The listing builds one solid part. Answer for the finished solid, in the listing's coordinates (mm). Face numbers are marked on the shaded views. A direction names the side the tool comes from. Round coordinates to 2 decimals unless told otherwise and drop trailing zeros. Order: outer loops, then holes, each group sorted by start corner. A loop starts at its lowest first (then second) coordinate and runs counter-clockwise, first axis right, second up. Notation, with made-up numbers: M -29.5,-20.5 L 19.5,-20.5 A30 cw 19.5,4.5 Z; hole C 17.5,18 d1. An arc over 180 degrees is marked long. Write item = value, one per line. Start each with the question number.
(1) A cutting plane is placed at D-D, the plane x = -10. Determine the outline of the cut face in (y, z), and give its area (3 significant figures).
(2) A cutting plane is placed at B-B, the plane z = -0.5. Determine the outline of the cut face in (x, y).
(3) Straight lines are drawn through the part: probe 1 along Z at (x, y) = (-4, 4.3); probe 2 along X at (y, z) = (0.55, 15); probe 3 along X at (y, z) = (3.45, -7) (3 decimals). For each, find the intervals that lie inside material, in ascending order. Write a range as from..to.
(4) A cutting plane is placed at C-C, the plane y = 4.25. Count the separate pieces of the cut face and the enclosed holes in it, and give its area (3 significant figures).
(5) A cutting plane is placed at A-A, the plane x = 8.5. Determine the outline of the cut face in (y, z) (3 decimals), and give its area (3 significant figures).
(6) Each of these flat-tipped pins is pushed along its axis until it touches: pin 1 (1.7 mm diameter, centred on x = 10, z = 4.5, fed in from +Y); pin 2 (1.7 mm diameter, centred on x = -13.5, z = 15.5, fed in from +Y). Where does it stop, or does it pass through?
(7) Which of the six approach directions +Z, -Z, +X, -X, +Y, -Y give full straight-line access (tool end or side, diameter ignored) to the marked faces 1, 2 and 3?
from build123d import *

# Parameters (mm, degrees)
SKETCH1_W           = 45
SKETCH1_H           = 45
SKETCH1_R           = 1.7
BOSS_EXTRUDE1_DEPTH = 5
SKETCH7_R           = 2.9
CUT_EXTRUDE6_DEPTH  = 3
SKETCH4_R           = 0.925
CUT_EXTRUDE3_DEPTH  = 33.210246817
SKETCH5_R           = 0.95
CUT_EXTRUDE4_DEPTH  = 33.210246817
LPATTERN1_COUNT     = 5
LPATTERN1_PITCH     = 5
FILLET1_R           = 1
CUT_EXTRUDE7_START  = -4
CUT_EXTRUDE7_DEPTH  = 4
FILLET2_R           = 3
CHAMFER2_SIZE       = 2
CUT_EXTRUDE8_DEPTH  = 33.210246817


with BuildPart() as part:
    # Sketch1 → Boss-Extrude1 (new body)
    with BuildSketch(Plane(origin=(0, 0, 0), x_dir=(1, 0, 0), z_dir=(0, 1, 0))):
        Rectangle(SKETCH1_W, SKETCH1_H)
        with Locations(Location((-15, 15, 0), (0, 0, 270))):
            Circle(SKETCH1_R, mode=Mode.SUBTRACT)
        with Locations(Location((-15, -15, 0), (0, 0, 270))):
            Circle(SKETCH1_R, mode=Mode.SUBTRACT)
        with Locations(Location((15, -15, 0), (0, 0, 90))):
            Circle(SKETCH1_R, mode=Mode.SUBTRACT)
        with Locations(Location((15, 15, 0), (0, 0, 90))):
            Circle(SKETCH1_R, mode=Mode.SUBTRACT)
    extrude(amount=BOSS_EXTRUDE1_DEPTH)

    # Sketch7 → Cut-Extrude6 (cut)
    with BuildSketch(Plane(origin=(0, 5, 0), x_dir=(1, 0, 0), z_dir=(0, 1, 0))):
        with Locations(Location((-15, 15, 0), (0, 0, 270))):
            Circle(SKETCH7_R)
        with Locations(Location((15, 15, 0), (0, 0, 270))):
            Circle(SKETCH7_R)
        with Locations(Location((-15, -15, 0), (0, 0, 270))):
            Circle(SKETCH7_R)
        with Locations(Location((15, -15, 0), (0, 0, 270))):
            Circle(SKETCH7_R)
    extrude(amount=-CUT_EXTRUDE6_DEPTH, mode=Mode.SUBTRACT)

    # Sketch4 → Cut-Extrude3 (cut, through all)
    with BuildSketch(Plane(origin=(0, 5, 0), x_dir=(1, 0, 0), z_dir=(0, 1, 0))):
        with Locations(Location((-6.5, 20, 0), (0, 0, 270))):
            Circle(SKETCH4_R)
        with Locations(Location((8.5, 7, 0), (0, 0, 270))):
            Circle(SKETCH4_R)
    extrude(amount=-CUT_EXTRUDE3_DEPTH, mode=Mode.SUBTRACT)

    # Sketch5 → Cut-Extrude4 (cut, through all)
    with BuildSketch(Plane(origin=(0, 5, 0), x_dir=(1, 0, 0), z_dir=(0, 1, 0))):
        with Locations(Location((-10, -19.5, 0), (0, 0, 270))):
            Circle(SKETCH5_R)
        with Locations(Location((10, -19.5, 0), (0, 0, 90))):
            Circle(SKETCH5_R)
    cut_extrude4 = extrude(amount=-CUT_EXTRUDE4_DEPTH, mode=Mode.SUBTRACT)

    # LPattern1: Cut-Extrude4 ×5
    with Locations(*[(0, 0, -i * LPATTERN1_PITCH) for i in range(1, LPATTERN1_COUNT)]):
        add(cut_extrude4, mode=Mode.SUBTRACT)

    # Fillet1
    fillet1_edges = [part.edges().sort_by_distance(p)[0] for p in [
        (22.5, 2.5, 22.5),
        (-22.5, 2.5, 22.5),
        (-22.5, 2.5, -22.5),
        (22.5, 2.5, -22.5),
    ]]
    fillet(fillet1_edges, radius=FILLET1_R)

    # Sketch8 → Cut-Extrude7 (cut)
    with BuildSketch(Plane(origin=(0, 5, 0), x_dir=(1, 0, 0), z_dir=(0, 1, 0)).offset(CUT_EXTRUDE7_START)):
        Polygon((-4.5, 21), (7.5, 21), (15.5, 21), (15.5, 19.5), (7.5, 19.5), (7.5, 15), (-4.5, 15), align=None)
    extrude(amount=CUT_EXTRUDE7_DEPTH, mode=Mode.SUBTRACT)

    # Fillet2
    fillet2_edges = [part.edges().sort_by_distance(p)[0] for p in [
        (15.5, 1, -20.25),
    ]]
    fillet(fillet2_edges, radius=FILLET2_R)

    # Chamfer2
    chamfer2_edges = [part.edges().sort_by_distance(p)[0] for p in [
        (7.5, 3, -19.5),
    ]]
    chamfer(chamfer2_edges, length=CHAMFER2_SIZE)

    # Sketch9 → Cut-Extrude8 (cut, through all)
    with BuildSketch(Plane(origin=(0, 5, 0), x_dir=(1, 0, 0), z_dir=(0, 1, 0))):
        with BuildLine():
            Line((-9, 22.5), (-9, 6.5))
            Line((-9, 6.5), (-22.5, -7))
            Line((-22.5, -7), (-22.5, 21.5))
            ThreePointArc((-22.5, 21.5), (-22.207106781, 22.207106781), (-21.5, 22.5))
            Line((-21.5, 22.5), (-9, 22.5))
        make_face()
        with BuildLine():
            Line((21.5, 22.5), (11, 22.5))
            Line((11, 22.5), (11, 4.5))
            Line((11, 4.5), (22.5, -7))
            Line((22.5, -7), (22.5, 21.5))
            ThreePointArc((22.5, 21.5), (22.207106781, 22.207106781), (21.5, 22.5))
        make_face()
    extrude(amount=-CUT_EXTRUDE8_DEPTH, mode=Mode.SUBTRACT)


solid = part.part
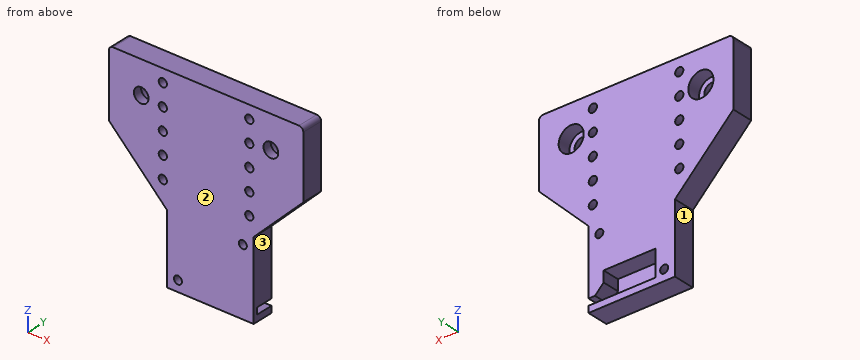
Reported:
q1.outline = M 0,-5.5 L 5,-5.5 L 5,-1.45 L 0,-1.45 Z; M 0,0.45 L 5,0.45 L 5,3.55 L 0,3.55 Z; M 0,5.45 L 5,5.45 L 5,8.55 L 0,8.55 Z; M 0,10.45 L 5,10.45 L 5,13.55 L 0,13.55 Z; M 0,15.45 L 5,15.45 L 5,18.55 L 0,18.55 Z; M 0,20.45 L 5,20.45 L 5,22.5 L 0,22.5 Z
q1.area = 92.5 mm²
q2.outline = M -15,0 L -10.95,0 L -10.95,5 L -15,5 Z; M -9.05,0 L 9.05,0 L 9.05,5 L -9.05,5 Z; M 10.95,0 L 15,0 L 15,5 L 10.95,5 Z
q3.probe_1 = -22.5..-21, -15..22.5
q3.probe_2 = -22.5..-16.7, -13.3..-10.81, -9.19..9.19, 10.81..13.3, 16.7..22.5
q3.probe_3 = -9..7.575, 9.425..11
q4.separate_pieces = 1
q4.enclosed_holes = 14
q4.area = 1,280 mm²
q5.outline = M 0,-22.5 L 5,-22.5 L 5,-21 L 1,-21 L 1,-18.5 L 5,-18.5 L 5,-7.925 L 0,-7.925 Z; M 0,-6.075 L 5,-6.075 L 5,22.5 L 0,22.5 Z
q5.area = 206 mm²
q6.pin_1 = through
q6.pin_2 = 2
q7.face_1 = -Z, -X, +Y, -Y
q7.face_2 = +Z, -Z, +X, -X, -Y
q7.face_3 = -Z, +X, +Y, -Y
